Design review of the part built by this model. Coordinates are the model's own, in mm. A direction names the side the tool comes from. Give positions to 0.01 mm unless a question says otherwise; leave off trailing zeros. Order: outer loops, then holes, each group sorted by start corner. A loop starts at its lowest first (then second) coordinate and runs counter-clockwise, first axis right, second up. Notation, with made-up numbers: (-17.75, 47) -> (24.25, 47) arc R22 cw to (24.25, 57) -> close; hole circle Ø1 at (19, 27). An arc over 180 degrees is marked (long way). One line per item, written item: value.
from build123d import *

# Parameters (mm, degrees)
SKETCH2_W           = 10
SKETCH2_H           = 10
BOSS_EXTRUDE1_DEPTH = 10
SKETCH3_R           = 5
BOSS_EXTRUDE2_DEPTH = 20
SKETCH4_W           = 16
SKETCH4_H           = 16
BOSS_EXTRUDE3_DEPTH = 10
SKETCH5_R           = 5
CUT_EXTRUDE1_DEPTH  = 4
SKETCH6_R           = 7
CUT_EXTRUDE2_DEPTH  = 4


with BuildPart() as part:
    # Sketch2 → Boss-Extrude1 (new body)
    with BuildSketch(Plane.XY):
        with Locations((5, -5)):
            Rectangle(SKETCH2_W, SKETCH2_H)
    boss_extrude1 = extrude(amount=BOSS_EXTRUDE1_DEPTH)

    # Sketch3 → Boss-Extrude2 (add)
    with BuildSketch(Plane(origin=(0, 0, 0), x_dir=(0, 0, -1), z_dir=(1, 0, 0))):
        with Locations(Location((-10, -5, 0), (0, 0, 90))):
            Circle(SKETCH3_R)
    boss_extrude2 = extrude(amount=BOSS_EXTRUDE2_DEPTH)

    # Mirror1: Boss-Extrude1, Boss-Extrude2 across plane
    add(boss_extrude1.mirror(Plane(origin=(0, 0, 10), x_dir=(0, 0, 1), z_dir=(1, 0, 0))))
    add(boss_extrude2.mirror(Plane(origin=(0, 0, 10), x_dir=(0, 0, 1), z_dir=(1, 0, 0))))

    # Sketch4 → Boss-Extrude3 (add)
    with BuildSketch(Plane(origin=(0, 0, 0), x_dir=(-1, 0, 0), z_dir=(0, 0, -1))):
        with Locations((0, -5)):
            Rectangle(SKETCH4_W, SKETCH4_H)
    extrude(amount=BOSS_EXTRUDE3_DEPTH)

    # Sketch5 → Cut-Extrude1 (cut)
    with BuildSketch(Plane(origin=(0, 0, -10), x_dir=(-1, 0, 0), z_dir=(0, 0, -1))):
        with Locations((0, -5)):
            Circle(SKETCH5_R)
    extrude(amount=-CUT_EXTRUDE1_DEPTH, mode=Mode.SUBTRACT)

    # Sketch6 → Cut-Extrude2 (cut)
    with BuildSketch(Plane(origin=(0, 0, -6), x_dir=(-1, 0, 0), z_dir=(0, 0, -1))):
        with Locations((0, -5)):
            Circle(SKETCH6_R)
    extrude(amount=-CUT_EXTRUDE2_DEPTH, mode=Mode.SUBTRACT)


solid = part.part
Item 1: Add section A-A on z = -3.5. Give the boundary of the cut face in (x, y).
Returned:
outline: (-8, -13) -> (8, -13) -> (8, 3) -> (-8, 3) -> close; hole circle Ø14 at (0, -5)
Item 2: Add section C-C on y = -5. Give the boundary of the cut face in (x, z).
Returned:
outline: (-20, 5) -> (-10, 5) -> (-10, 0) -> (-8, 0) -> (-8, -10) -> (-5, -10) -> (-5, -6) -> (-7, -6) -> (-7, -2) -> (7, -2) -> (7, -6) -> (5, -6) -> (5, -10) -> (8, -10) -> (8, 0) -> (10, 0) -> (10, 5) -> (20, 5) -> (20, 15) -> (-20, 15) -> close
Item 3: To check wall thickness, follow line 1 along Y through (x, z) = (0, -8.8); line 2 along Z through (x, y) = (-3, -11); line 3 along X through (y, z) = (2.25, -6). State the ranges of each line that lie inside material, in increasing order. Write a range as from..to.
Returned:
line 1: -13..-10, 0..3
line 2: -10..-6, -2..0
line 3: -8..8
Item 4: Add section D-D on y = 0.75. Give the boundary of the cut face in (x, z).
Returned:
outline: (-8, -10) -> (8, -10) -> (8, 0) -> (-8, 0) -> close; hole (-3.99, -6) -> (3.99, -6) -> (3.99, -2) -> (-3.99, -2) -> close
Item 5: Clearance check with flat-ended pins moving along their axes: P1, Ø0.6, axis at x = -9.5, y = -5, coming from the -Z side; P2, Ø3, axis at y = -2, z = 3.5, coming from the -X side; P3, Ø3, axis at y = 0.5, z = 0.5, coming from the +X side; P4, Ø8, axis at x = -13.5, z = -3.5, coming from the +Y side. State where each tip first meets the part, or that it passes through.
Returned:
P1: z = 0
P2: x = -10
P3: x = 10
P4: through
Item 6: Add section B-B on x = 7.5. Give the boundary of the cut face in (y, z), plus the area to 3 significant figures.
Returned:
outline: (-13, -10) -> (3, -10) -> (3, 0) -> (0, 0) -> (0, 10) arc R5 ccw to (-10, 10) -> (-10, 0) -> (-13, 0) -> close
area: 299 mm²
Item 7: Machinability: for faces 4 (the flat face through (-8, -5, -5)), 5 (the cylindrical face through (1.517, -11.834, -4.028)), 6 (the flat face through (9, -5, 0)), 7 (the cylindrical face through (4, -8, -8)), 8 (the flat face through (0, -10, 5)), which of the approach directions +Z, -Z, +X, -X, +Y, -Y give a long, thin tool a straight path to every point of the face, cutting with its end or side? Answer none if there is none.
Returned:
face 4: -Z, -X, +Y, -Y
face 5: none
face 6: -Z, +X, +Y, -Y
face 7: -Z
face 8: +Z, +X, -X, -Y
Item 8: Draft analysis for pull direction Z (two halves, no side actions). For faces 1 (the flat face through (0, -5, -2)), 2 (the flat face through (0, -11, 0)), 3 (the flat face through (0, 0, 5)), state which applies: pulls with the +Z half, pulls with the -Z half, needs draft (parallel to the pull), parting line crosses it, or undercut.
Returned:
face 1: undercut
face 2: pulls with the +Z half
face 3: needs draft
